Verification items for the finished model (mm, model axes). Face numbers are marked on the shaded views. Give positions to 0.01 mm unless a question says otherwise; leave off trailing zeros. Write each loop counter-clockwise with the first axis right and the second up, starting at its lowest first coordinate (ties: lowest second). Pieces come first, ordered by that corner, then holes. Notation, with made-up numbers: (-34, 26.5) - (-27, 26.5) arc R30 ccw to (-27, 54.5) - close; hole circle Ø11 at (80, -38). An arc over 180 degrees is marked (long way). Answer as a JSON object with one key per item and string values. Group by question number.
Item 1: Go/stop test with flat-tipped pins: pin 1 (8 mm diameter, centred on x = 44.5, z = -9.5, fed in from -Y); pin 2 (6 mm diameter, centred on x = 28, z = -13.5, fed in from -Y); pin 3 (3 mm diameter, centred on x = 44.5, y = -16, fed in from +Z). Record where each tip stops, or that it passes through.
Item 2: Scan lines: line 1 along Z through (x, y) = (33, -14); line 2 along Z through (x, y) = (22, -12); line 3 along Y through (x, z) = (32.5, -4.5). Record each from-to range of solid material in increasing order. Write a range as [from, to].
Item 3: Sectioned sample at A-A, the plane z = -9.75. Record the boundary of the cut face in (x, y).
Item 4: Sectioned sample at D-D, the plane y = -5.5. Record the boundary of the cut face in (x, z).
Item 5: Sectioned sample at C-C, the plane x = 34. Record the boundary of the cut face in (y, z), and give its area (3 significant figures).
Item 6: Draft check along Y on the marked faces 1, 2 and 3. Enter one of: +Y half, -Y half, draft (parallel to the pull), parting line (faces both ways), or undercut.
Item 7: Sectioned sample at B-B, the plane y = 7. Record the boundary of the cut face in (x, z), and give its area (3 significant figures).
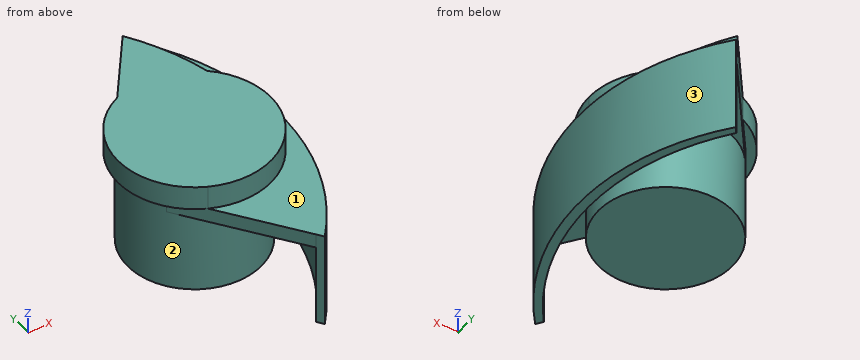
```python
from build123d import *

# Parameters (mm, degrees)
SKETCH3_R           = 14
BOSS_EXTRUDE1_DEPTH = 5
BOSS_EXTRUDE2_START = -3
SKETCH3_3_R         = 14
BOSS_EXTRUDE2_DEPTH = 3
BOSS_EXTRUDE3_START = -20
BOSS_EXTRUDE3_DEPTH = 20
BOSS_EXTRUDE4_START = -20
SKETCH3_5_R         = 14
BOSS_EXTRUDE4_DEPTH = 20
BOSS_EXTRUDE5_DEPTH = 5


with BuildPart() as part:
    # Sketch3 → Boss-Extrude1 (new body)
    with BuildSketch(Plane.XY):
        with Locations((32, 0)):
            Circle(SKETCH3_R)
    extrude(amount=BOSS_EXTRUDE1_DEPTH)

    # Sketch3_3 → Boss-Extrude2 (add)
    with BuildSketch(Plane.XY.offset(BOSS_EXTRUDE2_START)):
        with BuildLine():
            ThreePointArc((37.349918698, -30.84775354), (48, 0), (37.349918698, 30.84775354))
            Line((37.349918698, 30.84775354), (20.731628295, 8.308056278))
            ThreePointArc((20.731628295, 8.308056278), (36.372802084, 13.299571494), (46, 0))
            ThreePointArc((46, 0), (36.372802084, -13.299571494), (20.731628295, -8.308056278))
            Line((20.731628295, -8.308056278), (37.349918698, -30.84775354))
        make_face()
        with Locations(Location((32, 0, 0), (0, 0, 216.400975566))):
            Circle(SKETCH3_3_R)
        with BuildLine():
            ThreePointArc((38.302222156, -32.139380484), (50, 0), (38.302222156, 32.139380484))
            Line((38.302222156, 32.139380484), (37.349918698, 30.84775354))
            ThreePointArc((37.349918698, 30.84775354), (48, 0), (37.349918698, -30.84775354))
            Line((37.349918698, -30.84775354), (38.302222156, -32.139380484))
        make_face()
    extrude(amount=BOSS_EXTRUDE2_DEPTH)

    # Sketch3_4 → Boss-Extrude3 (add)
    with BuildSketch(Plane.XY.offset(BOSS_EXTRUDE3_START)):
        with BuildLine():
            ThreePointArc((38.302222156, -32.139380484), (50, 0), (38.302222156, 32.139380484))
            Line((38.302222156, 32.139380484), (37.349918698, 30.84775354))
            ThreePointArc((37.349918698, 30.84775354), (48, 0), (37.349918698, -30.84775354))
            Line((37.349918698, -30.84775354), (38.302222156, -32.139380484))
        make_face()
    extrude(amount=BOSS_EXTRUDE3_DEPTH)

    # Sketch3_5 → Boss-Extrude4 (add)
    with BuildSketch(Plane.XY.offset(BOSS_EXTRUDE4_START)):
        with Locations((32, 0)):
            Circle(SKETCH3_5_R)
    extrude(amount=BOSS_EXTRUDE4_DEPTH)

    # Sketch4 → Boss-Extrude5 (add)
    with BuildSketch(Plane.XY):
        with BuildLine():
            ThreePointArc((42.526315789, 12.049758334), (39.646765333, 20.405215379), (35.341109992, 28.123168822))
            Line((35.341109992, 28.123168822), (25.328337382, 14.542658557))
            ThreePointArc((25.328337382, 14.542658557), (34.295261564, 15.834512129), (42.526315789, 12.049758334))
        make_face()
        with BuildLine():
            Line((20.731628295, 8.308056278), (25.328337382, 14.542658557))
            ThreePointArc((25.328337382, 14.542658557), (16, 0), (25.328337382, -14.542658557))
            Line((25.328337382, -14.542658557), (20.731628295, -8.308056278))
            ThreePointArc((20.731628295, -8.308056278), (46, 0), (20.731628295, 8.308056278))
        make_face()
        with BuildLine():
            ThreePointArc((42.526315789, 12.049758334), (34.295261564, 15.834512129), (25.328337382, 14.542658557))
            Line((25.328337382, 14.542658557), (20.731628295, 8.308056278))
            ThreePointArc((20.731628295, 8.308056278), (46, 0), (20.731628295, -8.308056278))
            Line((20.731628295, -8.308056278), (25.328337382, -14.542658557))
            ThreePointArc((25.328337382, -14.542658557), (40.638674612, -13.467490521), (48, 0))
            ThreePointArc((48, 0), (46.567447488, 6.617361535), (42.526315789, 12.049758334))
        make_face()
    extrude(amount=BOSS_EXTRUDE5_DEPTH)


solid = part.part
```
Geometry check:
{
 "1": {"pin 1": "y = -29.32", "pin 2": "y = -13.96", "pin 3": "z = 0"},
 "2": {"line 1": "[-3, 5]", "line 2": "[0, 5]", "line 3": "[-13.99, 13.99]"},
 "3": {"outline": "circle Ø28 at (32, 0); (37.35, -30.85) - (38.3, -32.14) arc R50 ccw to (38.3, 32.14) - (37.35, 30.85) arc R50 cw to start"},
 "4": {"outline": "(16.98, 0) - (19.13, 0) - (19.13, -20) - (44.87, -20) - (44.87, -3) - (47.7, -3) - (47.7, -20) - (49.7, -20) - (49.7, 0) - (47.02, 0) - (47.02, 5) - (16.98, 5) - close"},
 "5": {"outline": "(-26.3, -3) - (-13.86, -3) - (-13.86, -20) - (13.86, -20) - (13.86, -3) - (26.3, -3) - (26.3, 5) - (-15.87, 5) - (-15.87, 0) - (-26.3, 0) - close", "area": "840 mm^2"},
 "6": {"face 1": "draft", "face 2": "undercut", "face 3": "parting line"},
 "7": {"outline": "(17.61, 0) - (19.88, 0) - (19.88, -20) - (44.12, -20) - (44.12, -3) - (47.51, -3) - (47.51, -20) - (49.51, -20) - (49.51, 0) - (46.39, 0) - (46.39, 5) - (17.61, 5) - close", "area": "679 mm^2"}
}
